Build history of the part. All positions in model axes, mm. Face numbers are marked on the shaded views. A direction names the side the tool comes from. Give positions to 0.01 mm unless a question says otherwise; leave off trailing zeros. Order: outer loops, then holes, each group sorted by start corner. A loop starts at its lowest first (then second) coordinate and runs counter-clockwise, first axis right, second up. Notation, with made-up numbers: M -36.75,23 L -32.75,23 A25 cw -32.75,60 Z; hole C -15.5,-31 d2. An arc over 180 degrees is marked long. One line per item, written item: value.
from build123d import *

# Parameters (mm, degrees)
SKETCH1_W           = 39
SKETCH1_H           = 13
BOSS_EXTRUDE1_DEPTH = 5
SKETCH5_W           = 39
SKETCH5_H           = 9
CUT_EXTRUDE1_DEPTH  = 2
SKETCH2_W           = 1
SKETCH2_H           = 9
BOSS_EXTRUDE2_DEPTH = 1
SKETCH6_R           = 1.65
CUT_EXTRUDE2_DEPTH  = 6
CHAMFER1_SIZE       = 1


with BuildPart() as part:
    # Sketch1 → Boss-Extrude1 (new body)
    with BuildSketch(Plane(origin=(0, 0, 0), x_dir=(1, 0, 0), z_dir=(0, 1, 0))):
        Rectangle(SKETCH1_W, SKETCH1_H)
    extrude(amount=BOSS_EXTRUDE1_DEPTH)

    # Sketch5 → Cut-Extrude1 (cut)
    with BuildSketch(Plane(origin=(0, 5, 0), x_dir=(1, 0, 0), z_dir=(0, 1, 0))):
        Rectangle(SKETCH5_W, SKETCH5_H)
    extrude(amount=-CUT_EXTRUDE1_DEPTH, mode=Mode.SUBTRACT)

    # Sketch2 → Boss-Extrude2 (add)
    with BuildSketch(Plane(origin=(0, 3, 0), x_dir=(1, 0, 0), z_dir=(0, 1, 0))):
        with Locations((7, 0)):
            Rectangle(SKETCH2_W, SKETCH2_H)
        with Locations((5, 0)):
            Rectangle(SKETCH2_W, SKETCH2_H)
        with Locations((9, 0)):
            Rectangle(SKETCH2_W, SKETCH2_H)
        with Locations((3, 0)):
            Rectangle(SKETCH2_W, SKETCH2_H)
        with Locations((11, 0)):
            Rectangle(SKETCH2_W, SKETCH2_H)
        with Locations((13, 0)):
            Rectangle(SKETCH2_W, SKETCH2_H)
        with Locations((15, 0)):
            Rectangle(SKETCH2_W, SKETCH2_H)
        with Locations((-3, 0)):
            Rectangle(SKETCH2_W, SKETCH2_H)
        with Locations((17, 0)):
            Rectangle(SKETCH2_W, SKETCH2_H)
        with Locations((-5, 0)):
            Rectangle(SKETCH2_W, SKETCH2_H)
        with Locations((19, 0)):
            Rectangle(SKETCH2_W, SKETCH2_H)
        with Locations((-7, 0)):
            Rectangle(SKETCH2_W, SKETCH2_H)
        with Locations((-9, 0)):
            Rectangle(SKETCH2_W, SKETCH2_H)
        with Locations((-11, 0)):
            Rectangle(SKETCH2_W, SKETCH2_H)
        with Locations((-13, 0)):
            Rectangle(SKETCH2_W, SKETCH2_H)
        with Locations((-15, 0)):
            Rectangle(SKETCH2_W, SKETCH2_H)
        with Locations((-17, 0)):
            Rectangle(SKETCH2_W, SKETCH2_H)
        with Locations((-19, 0)):
            Rectangle(SKETCH2_W, SKETCH2_H)
    extrude(amount=BOSS_EXTRUDE2_DEPTH)

    # Sketch6 → Cut-Extrude2 (cut, through all)
    with BuildSketch(Plane.XZ):
        Circle(SKETCH6_R)
    extrude(amount=-CUT_EXTRUDE2_DEPTH, mode=Mode.SUBTRACT)

    # Chamfer1
    chamfer1_edges = [part.edges().sort_by_distance(p)[0] for p in [
        (-19.5, 0, 0),
        (0, 0, -6.5),
        (19.5, 0, 0),
        (0, 0, 6.5),
    ]]
    chamfer(chamfer1_edges, length=CHAMFER1_SIZE)


solid = part.part
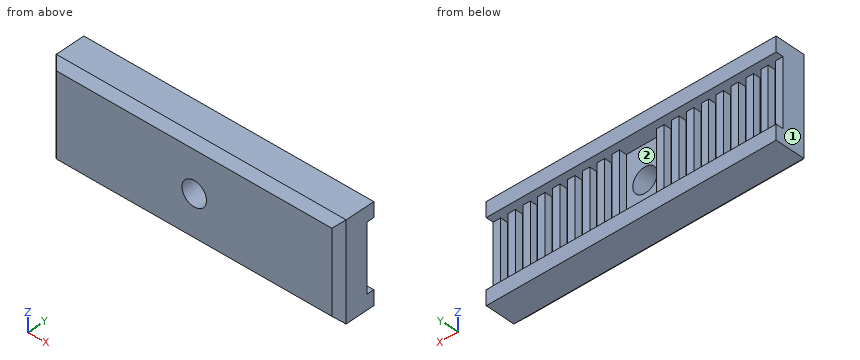
1) Saw through at D-D, the plane y = 3.55. Give the number of separate pieces and of enclosed holes in the cut face, then the cut area to 3 significant figures.
Check values:
separate pieces: 1
enclosed holes: 17
area: 318 mm^2
2) Saw through at A-A, the plane x = 0. Write the cut outline in (y, z), then the cut area to 3 significant figures.
Check values:
outline: M 0,-5.5 L 1,-6.5 L 5,-6.5 L 5,-4.5 L 3,-4.5 L 3,-1.65 L 0,-1.65 Z; M 0,1.65 L 3,1.65 L 3,4.5 L 5,4.5 L 5,6.5 L 1,6.5 L 0,5.5 Z
area: 36.1 mm^2
3) Pin check, flat tips, straight feed: pin 1 (0.5 mm diameter, centred on x = 13, z = -2, fed in from +Y); pin 2 (0.8 mm diameter, centred on x = 10, z = 0, fed in from +Y). Stop position of each tip, or through.
Check values:
pin 1: y = 4
pin 2: y = 3
4) Tool access for the marked faces 1 and 2: list every direction of +Z, -Z, +X, -X, +Y, -Y with a clear straight run to the whole face (end or side of a thin tool).
Check values:
face 1: +Z, -Z, -X, +Y, -Y
face 2: +Y
5) Saw through at C-C, the plane x = -14. Write the cut outline in (y, z), then the cut area to 3 significant figures.
Check values:
outline: M 0,-5.5 L 1,-6.5 L 5,-6.5 L 5,-4.5 L 3,-4.5 L 3,4.5 L 5,4.5 L 5,6.5 L 1,6.5 L 0,5.5 Z
area: 46.0 mm^2
6) Saw through at B-B, the plane y = 0.45. Write the cut outline in (x, z).
Check values:
outline: M -18.95,-5.95 L 18.95,-5.95 L 18.95,5.95 L -18.95,5.95 Z; hole C 0,0 d3.3
7) Drill centre lines: probe 1 along Z at (x, y) = (0, 2.25); probe 2 along Z at (x, y) = (-9, 4.45); probe 3 along Y at (x, z) = (-5, 2.25). Where is each one in solid material? Low to high. Write a range as from..to.
Check values:
probe 1: -6.5..-1.65, 1.65..6.5
probe 2: -6.5..-4.5, 4.5..6.5
probe 3: 0..4
